Check sheet for the modelled part. Datum: model origin and axes. Units: mm. A direction names the side the tool comes from. Give positions to 0.01 mm unless a question says otherwise; leave off trailing zeros. Order: outer loops, then holes, each group sorted by start corner. A loop starts at its lowest first (then second) coordinate and runs counter-clockwise, first axis right, second up. Notation, with made-up numbers: (64, -18) -> (68, -18) arc R24 cw to (68, 11) -> close; hole circle Ø4 at (-0.75, -29.5). An arc over 180 degrees is marked (long way). Answer in a Markdown table with one row per item. Add a question column.
(1) Cross-section at A-A (x = 103). Record the cut outline in (y, z), then the cut area to 3 significant figures.
(2) Cross-section at D-D (x = 33.5). Record the cut outline in (y, z).
(3) Release check for a two-part mould opening along Y. For faces 1 (the face through (-2, 950, 0)), 2 (the face through (5.331, -930.734, 149.905)), 3 (the face through (-1, -912, 1)) record: released by +Y, released by -Y, zero draft, split by the parting line, or undercut.
(4) Cross-section at B-B (z = 0). Record the cut outline in (x, y), then the cut area to 3 significant figures.
(5) Thickness scan on L1, parallel to Y at x = 52, z = -123.5; L2, parallel to Z at x = 0, y = -356; L3, parallel to X at y = 727, z = 31.5. Record the ranges inside material, lowest first. Write a range as [from, to].
(6) Go/stop test with flat-tipped pins: pin 1 (1.5 mm diameter, centred on x = -17, y = -598.5, fed in from +Z); pin 2 (15.5 mm diameter, centred on y = -937.5, z = -131.5, fed in from -X); pin 3 (25 mm diameter, centred on y = 937.5, z = -142.5, fed in from +X); pin 4 (23 mm diameter, centred on x = 0, z = -110, fed in from -Y). Record where each tip stops, or that it passes through.
(7) Cross-section at C-C (y = 214). Record the cut outline in (x, z), then the cut area to 3 significant figures.
(8) Set-up check for faces 4 (the face through (80.312, -12.768, 25.291)), 5 (the face through (-85, 931, -139)), 6 (the face through (85, -931, -140)): record each of +Z, -Z, +X, -X, +Y, -Y from which the full face is reachable in a straight line by a thin tool's end or side.
```python
from build123d import *

# Parameters (mm, degrees)
F0_R      = 84.2
F0_R_2    = 76.2
F1_DEPTH  = 912
F2_R      = 75
F3_DEPTH  = 10
F4_R      = 10
F5_DEPTH  = 10
F8_DEPTH  = 38
F9_R      = 10
F10_DEPTH = 38


# Not quite as in the source:
# - a pattern or mirror of a feature is missing from the dataset's text; its kind, count and spacing are read off the source's solid
# - a feature names something its author has since deleted; it is built from what else it names


with BuildPart() as f1:
    # F0 (on Front) → F1 (new body, symmetric)
    with BuildSketch(Plane.XZ):
        Circle(F0_R)
        Circle(F0_R_2, mode=Mode.SUBTRACT)
    extrude(amount=F1_DEPTH, both=True)

    # F7 (on face) → F8 (join)
    with BuildSketch(Plane.XZ.offset(912)):
        with BuildLine():
            Line((85, -155), (85, -123.5920709431))
            ThreePointArc((85, -123.5920709431), (0, 150), (-85, -123.5920709431))
            Line((-85, -123.5920709431), (-85, -155))
            Line((-85, -155), (85, -155))
        make_face()
    f8 = extrude(amount=F8_DEPTH)

    # F8_copies: F8 across plane
    add(f8.mirror(Plane.ZX))

    # F9 (on face) → F10 (cut, through all)
    with BuildSketch(Plane.XZ.offset(950)):
        with Locations((-70.7066370655, 84.2648887431)):
            Circle(F9_R)
        with Locations((0, 110)):
            Circle(F9_R)
        with Locations((70.7066370655, 84.2648887431)):
            Circle(F9_R)
        with Locations((-70.7066370655, -84.2648887431)):
            Circle(F9_R)
        with Locations((0, -110)):
            Circle(F9_R)
        with Locations((70.7066370655, -84.2648887431)):
            Circle(F9_R)
    f10 = extrude(amount=-F10_DEPTH, mode=Mode.SUBTRACT)

    # F10_copies: F10 across plane
    add(f10.mirror(Plane.ZX), mode=Mode.SUBTRACT)


with BuildPart() as f3:
    # F2 (on face) → F3 (new body)
    with BuildSketch(Plane.XZ.offset(912)):
        Circle(F2_R)
    extrude(amount=F3_DEPTH)

    # F4 (on face) → F5 (cut, through all)
    with BuildSketch(Plane.XZ.offset(922)):
        with Locations((0, 61)):
            Circle(F4_R)
        with Locations((-52.8275496309, 30.5)):
            Circle(F4_R)
        with Locations((-52.8275496309, -30.5)):
            Circle(F4_R)
        with Locations((0, -61)):
            Circle(F4_R)
        with Locations((52.8275496309, -30.5)):
            Circle(F4_R)
        with Locations((52.8275496309, 30.5)):
            Circle(F4_R)
    extrude(amount=-F5_DEPTH, mode=Mode.SUBTRACT)


solid = f1.part
```
Answer below:
| question | item | result |
|---|---|---|
| 1 | outline | (-950, -109.05) -> (-912, -109.05) -> (-912, 109.05) -> (-950, 109.05) -> close; (912, -109.05) -> (950, -109.05) -> (950, 109.05) -> (912, 109.05) -> close |
| 1 | area | 16,600 mm² |
| 2 | outline | (-950, -155) -> (-912, -155) -> (-912, -77.25) -> (912, -77.25) -> (912, -155) -> (950, -155) -> (950, 146.21) -> (912, 146.21) -> (912, 77.25) -> (-912, 77.25) -> (-912, 146.21) -> (-950, 146.21) -> close; hole (-912, -68.44) -> (912, -68.44) -> (912, 68.44) -> (-912, 68.44) -> close |
| 3 | face 1 | released by +Y |
| 3 | face 2 | zero draft |
| 3 | face 3 | undercut |
| 4 | outline | (-150, -950) -> (150, -950) -> (150, -912) -> (84.2, -912) -> (84.2, 912) -> (150, 912) -> (150, 950) -> (-150, 950) -> (-150, 912) -> (-84.2, 912) -> (-84.2, -912) -> (-150, -912) -> close; hole (-76.2, -912) -> (76.2, -912) -> (76.2, 912) -> (-76.2, 912) -> close |
| 4 | area | 52,000 mm² |
| 5 | L1 | y = [-950, -912], [912, 950] |
| 5 | L2 | z = [-84.2, -76.2], [76.2, 84.2] |
| 5 | L3 | x = [-78.09, -69.38], [69.38, 78.09] |
| 6 | pin 1 | stops at z = 82.62 |
| 6 | pin 2 | stops at x = -85 |
| 6 | pin 3 | stops at x = 85 |
| 6 | pin 4 | stops at y = -950 |
| 7 | outline | circle Ø168.4 at (0, 0); hole circle Ø152.4 at (0, 0) |
| 7 | area | 4,030 mm² |
| 8 | face 4 | none |
| 8 | face 5 | -Z, -X, +Y, -Y |
| 8 | face 6 | -Z, +X, +Y, -Y |
